```python
from build123d import *

# Parameters (mm, degrees)
SKETCH1_W           = 44
SKETCH1_H           = 17
BOSS_EXTRUDE1_DEPTH = 12
FILLET1_R           = 1
SKETCH2_W           = 40
SKETCH2_H           = 13
BOSS_EXTRUDE2_DEPTH = 0.6


with BuildPart() as part:
    # Sketch1 → Boss-Extrude1 (new body)
    with BuildSketch(Plane(origin=(0, 0, 0), x_dir=(1, 0, 0), z_dir=(0, 1, 0))):
        Rectangle(SKETCH1_W, SKETCH1_H)
    extrude(amount=BOSS_EXTRUDE1_DEPTH)

    # Fillet1
    fillet1_edges = [part.edges().sort_by_distance(p)[0] for p in [
        (-22, 12, 0),
        (0, 12, 8.5),
        (22, 12, 0),
        (0, 0, 8.5),
        (-22, 0, 0),
        (0, 0, -8.5),
        (22, 0, 0),
        (22, 6, 8.5),
        (-22, 6, 8.5),
        (-22, 6, -8.5),
        (22, 6, -8.5),
        (0, 12, -8.5),
    ]]
    fillet(fillet1_edges, radius=FILLET1_R)

    # Sketch2 → Boss-Extrude2 (add)
    with BuildSketch(Plane.XZ):
        Rectangle(SKETCH2_W, SKETCH2_H)
    extrude(amount=BOSS_EXTRUDE2_DEPTH)


solid = part.part
```
Design review of the part built by this model. Coordinates are the model's own, in mm. Coordinates: 2 decimals unless noted, no trailing zeros. Loops run counter-clockwise (first coordinate to the right, second up) from the corner with the lowest first, then second, coordinate; pieces in that order, holes last. Notation, with made-up numbers: (0.25, 77) - (34.25, 77) arc R13 cw to (34.25, 102) - close; hole circle Ø4 at (-38, 17.25). An arc over 180 degrees is marked (long way). Use CSV: the item, a comma, the result in double quotes. Start each with the question number.
1) Wall thickness on L1, parallel to Y at x = 16.5, z = 7.5; L2, parallel to X at y = 11.5, z = 5; L3, parallel to X at y = 0.25, z = 5.75: over which ranges is each line inside the solid? List them lowest first. Write a range as from..to.
2) Consider section B-B on z = 7. Write out the cut boundary in (x, y), then the cut area to 3 significant figures.
3) For pin 1 Ø0.7 at (x, y) = (-9.5, 0) entering from +Z; pin 2 Ø0.7 at (y, z) = (-0.5, 2.5) entering from +X, all flat-tipped, find the tip position at first contact; note any pin that passes through.
4) Consider section A-A on x = -16.5. Write out the cut boundary in (y, z).
Geometry says:
1,L1,"0..12"
1,L2,"-21.87..21.87"
1,L3,"-21.66..21.66"
2,outline,"(-22, 1) arc R1 ccw to (-21, 0) - (21, 0) arc R1 ccw to (22, 1) - (22, 11) arc R1 ccw to (21, 12) - (-21, 12) arc R1 ccw to (-22, 11) - close"
2,area,"527 mm^2"
3,pin 1,"z = 8.26"
3,pin 2,"x = 20"
4,outline,"(-0.6, -6.5) - (0, -6.5) - (0, -7.5) arc R1 ccw to (1, -8.5) - (11, -8.5) arc R1 ccw to (12, -7.5) - (12, 7.5) arc R1 ccw to (11, 8.5) - (1, 8.5) arc R1 ccw to (0, 7.5) - (0, 6.5) - (-0.6, 6.5) - close"
